Design review of the part built by this model. Coordinates are the model's own, in mm. Coordinates: 2 decimals unless noted, no trailing zeros. Write each loop counter-clockwise with the first axis right and the second up, starting at its lowest first coordinate (ties: lowest second). Pieces come first, ordered by that corner, then holes.
Q1. For pin 1 Ø2 at (y, z) = (2, -40) entering from +X; pin 2 Ø1 at (x, y) = (61, 2.5) entering from +Z; pin 3 Ø1.5 at (y, z) = (3.5, -43) entering from -X, all flat-tipped, find the tip position at first contact; note any pin that passes through.
Q2. For L1, parallel to X at y = 5.5, z = -22; L2, parallel to X at y = 9, z = -9; L3, parallel to Z at x = 57.5, y = 3.5, list the stretches that pass through material, from the lowest coordinate up.
Q3. The part is to be moulded in two halves that separate along Z. For faces 1 (the cylindrical face through (44.57, 5.92, -3.06)), 2 (the cylindrical face through (47.84, 5.92, -7.82)), 3 (the flat face through (38, 12, -30)), say which applies: released by +Z, released by -Z, zero draft, split by the parting line, or undercut.
Q4. Take a section at C-C, the plane x = 25. Write out the cut boundary in (y, z), plus the area to 3 significant figures.
Q5. Take a section at D-D, the plane x = 50. Write out the cut boundary in (y, z).
Q6. Take a section at A-A, the plane x = 64. Write out the cut boundary in (y, z), plus the area to 3 significant figures.
Q7. Take a section at B-B, the plane z = -11. Write out the cut boundary in (x, y).
from build123d import *

# Parameters (mm, degrees)
SKETCH1_R           = 2.5
BOSS_EXTRUDE2_DEPTH = 12


with BuildPart() as part:
    # Sketch1 → Boss-Extrude2 (new body)
    with BuildSketch(Plane(origin=(0, 0, 0), x_dir=(1, 0, 0), z_dir=(0, 1, 0))):
        with BuildLine():
            ThreePointArc((45.159534103, 57.054132786), (44.573597006, 57.060491355), (43.987659909, 57.054132786))
            ThreePointArc((43.987659909, 57.054132786), (41.29051652, 52.222505932), (41.929927551, 46.72611129))
            ThreePointArc((41.929927551, 46.72611129), (39.359244243, 46.108619011), (36.916564905, 45.097171022))
            ThreePointArc((36.916564905, 45.097171022), (34.203159585, 49.919684069), (29.181165736, 52.243211197))
            ThreePointArc((29.181165736, 52.243211197), (28.703395194, 51.903950203), (28.233099598, 51.554400828))
            ThreePointArc((28.233099598, 51.554400828), (28.891023769, 46.060191485), (32.639017871, 41.989351186))
            ThreePointArc((32.639017871, 41.989351186), (30.922244243, 39.978779702), (29.540589358, 37.724730199))
            ThreePointArc((29.540589358, 37.724730199), (24.510796293, 40.031325579), (19.082182945, 38.959244591))
            ThreePointArc((19.082182945, 38.959244591), (18.895071066, 38.403950203), (18.720053904, 37.844726003))
            ThreePointArc((18.720053904, 37.844726003), (22.481740965, 33.786535398), (27.90671178, 32.696172074))
            ThreePointArc((27.90671178, 32.696172074), (27.699597006, 30.060491355), (27.90671178, 27.424810636))
            ThreePointArc((27.90671178, 27.424810636), (22.481740964, 26.334447311), (18.720053904, 22.276256707))
            ThreePointArc((18.720053904, 22.276256707), (18.895071066, 21.717032507), (19.082182945, 21.161738118))
            ThreePointArc((19.082182945, 21.161738118), (24.510796293, 20.089657131), (29.540589358, 22.396252511))
            ThreePointArc((29.540589358, 22.396252511), (30.922244243, 20.142203008), (32.639017871, 18.131631524))
            ThreePointArc((32.639017871, 18.131631524), (28.891023769, 14.060791225), (28.233099598, 8.566581881))
            ThreePointArc((28.233099598, 8.566581881), (28.703395194, 8.217032507), (29.181165736, 7.877771512))
            ThreePointArc((29.181165736, 7.877771512), (34.203159585, 10.20129864), (36.916564905, 15.023811688))
            ThreePointArc((36.916564905, 15.023811688), (39.359244243, 14.012363699), (41.929927551, 13.39487142))
            ThreePointArc((41.929927551, 13.39487142), (41.29051652, 7.898476778), (43.987659909, 3.066849924))
            ThreePointArc((43.987659909, 3.066849924), (44.573597006, 3.060491355), (45.159534103, 3.066849924))
            ThreePointArc((45.159534103, 3.066849924), (47.856677493, 7.898476778), (47.217266462, 13.39487142))
            ThreePointArc((47.217266462, 13.39487142), (49.787949769, 14.012363699), (52.230629107, 15.023811688))
            ThreePointArc((52.230629107, 15.023811688), (54.944034428, 10.201298641), (59.966028276, 7.877771513))
            ThreePointArc((59.966028276, 7.877771513), (60.443798818, 8.217032507), (60.914094414, 8.566581881))
            ThreePointArc((60.914094414, 8.566581881), (60.256170243, 14.060791225), (56.508176141, 18.131631524))
            ThreePointArc((56.508176141, 18.131631524), (58.224949769, 20.142203008), (59.606604654, 22.396252511))
            ThreePointArc((59.606604654, 22.396252511), (64.636397719, 20.089657131), (70.065011067, 21.161738118))
            ThreePointArc((70.065011067, 21.161738118), (70.252122946, 21.717032507), (70.427140109, 22.276256707))
            ThreePointArc((70.427140109, 22.276256707), (66.665453048, 26.334447311), (61.240482233, 27.424810636))
            ThreePointArc((61.240482233, 27.424810636), (61.447597006, 30.060491355), (61.240482233, 32.696172074))
            ThreePointArc((61.240482233, 32.696172074), (66.665453048, 33.786535398), (70.427140109, 37.844726003))
            ThreePointArc((70.427140109, 37.844726003), (70.252122946, 38.403950203), (70.065011067, 38.959244591))
            ThreePointArc((70.065011067, 38.959244591), (64.636397719, 40.031325579), (59.606604654, 37.724730199))
            ThreePointArc((59.606604654, 37.724730199), (58.224949769, 39.978779702), (56.508176141, 41.989351186))
            ThreePointArc((56.508176141, 41.989351186), (60.256170243, 46.060191485), (60.914094414, 51.554400828))
            ThreePointArc((60.914094414, 51.554400828), (60.443798818, 51.903950203), (59.966028276, 52.243211197))
            ThreePointArc((59.966028276, 52.243211197), (54.944034428, 49.919684069), (52.230629107, 45.097171022))
            ThreePointArc((52.230629107, 45.097171022), (49.787949769, 46.108619011), (47.217266462, 46.72611129))
            ThreePointArc((47.217266462, 46.72611129), (47.856677493, 52.222505932), (45.159534103, 57.054132786))
        make_face()
        with Locations(Location((44.573597006, 30.060491355, 0), (0, 0, 270))):  # turned: the seam where the file's is
            Circle(SKETCH1_R, mode=Mode.SUBTRACT)
    extrude(amount=BOSS_EXTRUDE2_DEPTH)


solid = part.part
Responses:
1. pin 1: stops at x = 69.99
1. pin 2: stops at z = -8.26
1. pin 3: stops at x = 30.43
2. L1: x = 18.8 to 29.08, 29.75 to 59.4, 60.07 to 70.34
2. L2: x = 28.16 to 32.56, 41.14 to 48.01, 56.58 to 60.99
2. L3: z = -51.58 to -42.64, -40.91 to -19.21, -17.48 to -8.54
3. face 1: released by +Z
3. face 2: undercut
3. face 3: zero draft
4. outline: (0, -39.96) - (12, -39.96) - (12, -32.84) - (0, -32.84) - close; (0, -27.28) - (12, -27.28) - (12, -20.16) - (0, -20.16) - close
4. area: 171 mm2
5. outline: (0, -46.04) - (12, -46.04) - (12, -14.08) - (0, -14.08) - close
6. outline: (0, -39.93) - (12, -39.93) - (12, -32.81) - (0, -32.81) - close; (0, -27.31) - (12, -27.31) - (12, -20.19) - (0, -20.19) - close
6. area: 171 mm2
7. outline: (28.09, 0) - (34.97, 0) - (34.97, 12) - (28.09, 12) - close; (41.22, 0) - (47.93, 0) - (47.93, 12) - (41.22, 12) - close; (54.18, 0) - (61.05, 0) - (61.05, 12) - (54.18, 12) - close
